```python
from build123d import *

# Parameters (mm, degrees)
F1_DEPTH = 60
F0_W     = 30
F0_H     = 60
F2_DEPTH = 10
F0_W_2   = 20
F0_H_2   = 40
F3_DEPTH = 30


with BuildPart() as f1:
    # F0 (on Front) → F1 (new body)
    with BuildSketch(Plane.XZ):
        Polygon((15, -30), (15, 30), (-25, 30), (-25, -10), (-45, -10), (-45, -30), (-35, -30), (-35, -20), (5, -20), (5, -30), align=None)
    extrude(amount=F1_DEPTH)

    # F0 (on Front) → F2 (join)
    with BuildSketch(Plane.XZ):
        with Locations((30, 0)):
            Rectangle(F0_W, F0_H)
    extrude(amount=F2_DEPTH)

    # F0 (on Front) → F3 (join)
    with BuildSketch(Plane.XZ):
        with Locations((-35, 10)):
            Rectangle(F0_W_2, F0_H_2)
    extrude(amount=F3_DEPTH)


solid = f1.part
```
Geometry check sheet. Reference: the model listing, model coordinates, mm. A direction names the side the tool comes from. Give positions to 0.01 mm unless a question says otherwise; leave off trailing zeros. Order: outer loops, then holes, each group sorted by start corner. A loop starts at its lowest first (then second) coordinate and runs counter-clockwise, first axis right, second up. Notation, with made-up numbers: (71.25, 86) -> (79.25, 86) arc R28 ccw to (79.25, 107) -> close; hole circle Ø4 at (-9, 13). An arc over 180 degrees is marked (long way). Write each question's results on one line, items separated by ' | '. Start each with the question number.
(1) Access from +Z, -Z, +X, -X, +Y, -Y to the whole of each face (thin tool, end or side, straight path). Record for faces 5 (the face through (-35, -30, 10)), 6 (the face through (5, -30, -25)), 7 (the face through (15, -35, 0)).
(2) Sectioned sample at A-A (y = -37). Enter the section's corners in (x, z), plus the area to 3 significant figures.
(3) Gauge pin test, flat ends, axial feed: P1, Ø1, axis at x = -30, z = 6, coming from the -Y side; P2, Ø15, axis at y = -52, z = 16, coming from the -X side; P3, Ø3, axis at x = 18.5, z = 0, coming from the +Y side; P4, Ø8, axis at y = -41, z = 3.5, coming from the +X side. Record the tip position at first contact, or that the pin passes through.
(4) Mould release check, pull along X, two halves, no side actions. Record for faces 1 (the face through (-1, 0, 0)), 2 (the face through (-45, -23, -7)), 3 (the face through (-15, -30, -20)), 4 (the face through (45, -5, 0)): pulls with the +X half, pulls with the -X half, needs draft (parallel to the pull), parting line crosses it, or undercut.
(5) Sectioned sample at C-C (x = -3). Enter the section's corners in (y, z).
(6) Sectioned sample at D-D (y = -28.5). Enter the section's corners in (x, z).
(7) Scan lines: line 1 (X direction, y = -37, z = -7.5); line 2 (Y direction, x = 16, z = 17.5); line 3 (Z direction, x = 2.5, y = -15). Record each from-to range of solid material in increasing order.
(8) Sectioned sample at B-B (z = -16.5). Enter the section's corners in (x, y).
Answer below:
1) face 5: +Z, -X, -Y | face 6: -Z, +Y, -Y | face 7: +Z, -Z, +X, -Y
2) outline: (-45, -30) -> (-35, -30) -> (-35, -20) -> (5, -20) -> (5, -30) -> (15, -30) -> (15, 30) -> (-25, 30) -> (-25, -10) -> (-45, -10) -> close | area: 2,400 mm2
3) P1: y = -30 | P2: x = -25 | P3: y = 0 | P4: x = 15
4) face 1: needs draft | face 2: pulls with the -X half | face 3: undercut | face 4: pulls with the +X half
5) outline: (-60, -20) -> (0, -20) -> (0, 30) -> (-60, 30) -> close
6) outline: (-45, -30) -> (-35, -30) -> (-35, -20) -> (5, -20) -> (5, -30) -> (15, -30) -> (15, 30) -> (-45, 30) -> close
7) line 1: -25 to 15 | line 2: -10 to 0 | line 3: -20 to 30
8) outline: (-45, -60) -> (15, -60) -> (15, -10) -> (45, -10) -> (45, 0) -> (-45, 0) -> close
